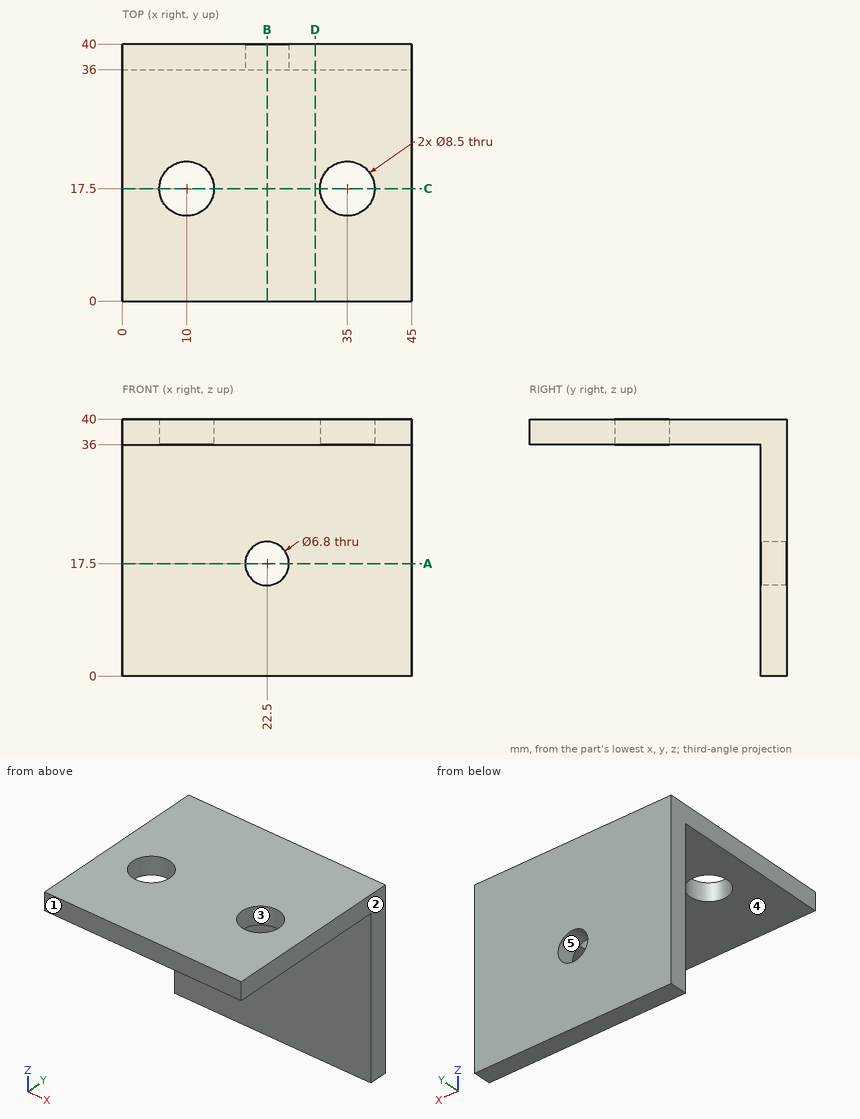
Drawing for the job (mm, zero at the part's lowest x, y, z). A direction names the side the tool comes from. Round coordinates to 2 decimals unless told otherwise and drop trailing zeros. Loops run counter-clockwise (first coordinate to the right, second up) from the corner with the lowest first, then second, coordinate; pieces in that order, holes last. Notation, with made-up numbers: M -33,20 L 22,20 A10 ccw 22,25 Z; hole C 57,57.25 d11. An arc over 180 degrees is marked long. Use a Markdown table: item, result. Add a question column.
(1) Which spindle directions (+Z, -Z, +X, -X, +Y, -Y) get a long thin tool onto all of the face, cutting with end or side? Do the marked faces 4 and 5. Say none if no direction does.
(2) Cut at B-B (x = 22.5). Give the cut face in (y, z), and give its area (3 significant figures).
(3) Pull direction X, two halves, no side cores. Call the marked faces 1, 2 and 3: +X half, -X half, draft (parallel to the pull), parting line (faces both ways), or undercut.
(4) Flat gauge pins, fed straight in: pin 1 (2 mm diameter, centred on x = 17.5, z = 33, fed in from -Y); pin 2 (11 mm diameter, centred on x = 21, y = 20.5, fed in from -Z). Where does each tip first touch, or does it go through?
(5) Cut at A-A (z = 17.5). Give the cut face in (x, y), and give its area (3 significant figures).
(6) Cut at C-C (y = 17.5). Give the cut face in (x, z), and give its area (3 significant figures).
(7) Drill centre lines: line 1 (Y direction, x = 10, z = 37); line 2 (X direction, y = 17, z = 38); line 3 (Z direction, x = 34.5, y = 33.5). Where is each one in solid material? Low to high.
(8) Cut at D-D (x = 30). Give the cut face in (y, z), and give its area (3 significant figures).
Geometry says:
| question | item | result |
|---|---|---|
| 1 | face 4 | -Z, +X, -X, -Y |
| 1 | face 5 | +Y, -Y |
| 2 | outline | M 0,36 L 36,36 L 36,20.9 L 40,20.9 L 40,40 L 0,40 Z; M 36,0 L 40,0 L 40,14.1 L 36,14.1 Z |
| 2 | area | 277 mm² |
| 3 | face 1 | draft |
| 3 | face 2 | +X half |
| 3 | face 3 | undercut |
| 4 | pin 1 | stops at y = 36 |
| 4 | pin 2 | stops at z = 36 |
| 5 | outline | M 0,36 L 19.1,36 L 19.1,40 L 0,40 Z; M 25.9,36 L 45,36 L 45,40 L 25.9,40 Z |
| 5 | area | 153 mm² |
| 6 | outline | M 0,36 L 5.75,36 L 5.75,40 L 0,40 Z; M 14.25,36 L 30.75,36 L 30.75,40 L 14.25,40 Z; M 39.25,36 L 45,36 L 45,40 L 39.25,40 Z |
| 6 | area | 112 mm² |
| 7 | line 1 | y = 0 to 13.25, 21.75 to 40 |
| 7 | line 2 | x = 0 to 5.78, 14.22 to 30.78, 39.22 to 45 |
| 7 | line 3 | z = 36 to 40 |
| 8 | outline | M 0,36 L 36,36 L 36,0 L 40,0 L 40,40 L 0,40 Z |
| 8 | area | 304 mm² |
